Read the model definition and answer for the solid it produces. Units are mm, in the model's axes. A direction names the side the tool comes from. Coordinates: 2 decimals unless noted, no trailing zeros. Write each loop counter-clockwise with the first axis right and the second up, starting at its lowest first coordinate (ties: lowest second). Pieces come first, ordered by that corner, then holes. Notation, with made-up numbers: (-15, 55) -> (1, 55) arc R19 ccw to (1, 72) -> close; hole circle Ø5 at (76.25, 55). An arc over 180 degrees is marked (long way). Write item = value, one per line. Start each with the question number.
1) For a pull along Z with two mould halves and no side action, classify faces 3 (the face through (225, -9, 114.3)), 4 (the face through (196.875, -9.658, 51.917)), 5 (the face through (135, -9, 0)) as released by +Z, released by -Z, zero draft, split by the parting line, or undercut.
2) A tool of negligible diameter and unlimited length cuts with its end or side. For faces 1 (the face through (136, -10, 50.8)), 2 (the face through (273.05, -9, 56)), from which of +Z, -Z, +X, -X, +Y, -Y can it reach the whole face along a straight path? Write none if from no direction.
3) Find the intervals of material crossed by line 1 along Z through (x, y) = (222.25, -9.5); line 2 along X through (y, z) = (-10.25, 106.5); line 3 along X through (y, z) = (-11, 37.5), in increasing order. Write a range as from..to.
4) Flat-ended cylindrical pins translate along their axes: pin 1 Ø4 at (x, y) = (189.5, -2.5) entering from -Z; pin 2 Ø9.5 at (x, y) = (123, -10.5) entering from +Z. Find the tip coordinate at first contact, or state that the pin passes through.
5) Section B-B (y = -14) is taken. Determine the outline of the cut face in (x, z) (3 decimals).
6) Section D-D (z = 30) is taken. Determine the outline of the cut face in (x, y).
7) Section A-A (x = 222.25) is taken. Determine the outline of the cut face in (y, z).
8) Section C-C (z = 85) is taken. Determine the outline of the cut face in (x, y), plus the area to 3 significant figures.
from build123d import *

# Parameters (mm, degrees)
F0_W     = 273.05
F0_H     = 114.3
F1_DEPTH = 19.05
F2_R     = 25.4
F3_DEPTH = 25.4
F5_DEPTH = 25.4


with BuildPart() as f1:
    # F0 (on Front) → F1 (new body)
    with BuildSketch(Plane.XZ):
        with Locations((136.525, 57.15)):
            Rectangle(F0_W, F0_H)
    extrude(amount=F1_DEPTH)

    # F2 (on face) → F3 (cut)
    with BuildSketch(Plane.XZ.offset(19.05)):
        with Locations((50.8, 50.8)):
            Circle(F2_R)
        with Locations((222.25, 50.8)):
            Circle(F2_R)
    extrude(amount=-F3_DEPTH, mode=Mode.SUBTRACT)

    # F4 (on face) → F5 (cut)
    with BuildSketch(Plane.XZ.offset(19.05)):
        with BuildLine():
            Line((177.8, 114.3), (95.25, 114.3))
            Line((95.25, 114.3), (95.25, 60.325))
            ThreePointArc((95.25, 60.325), (98.039808, 53.589808), (104.775, 50.8))
            Line((104.775, 50.8), (168.275, 50.8))
            ThreePointArc((168.275, 50.8), (175.010192, 53.589808), (177.8, 60.325))
            Line((177.8, 60.325), (177.8, 114.3))
        make_face()
    extrude(amount=-F5_DEPTH, mode=Mode.SUBTRACT)


solid = f1.part
Answer key:
q1.face_3 = released by +Z
q1.face_4 = undercut
q1.face_5 = released by -Z
q2.face_1 = +Z, +Y, -Y
q2.face_2 = +Z, -Z, +X, +Y, -Y
q3.line_1 = 0..25.4, 76.2..114.3
q3.line_2 = 0..95.25, 177.8..273.05
q3.line_3 = 0..29.16, 72.44..200.61, 243.89..273.05
q4.pin_1 = 0
q4.pin_2 = 50.8
q5.outline = (0, 0) -> (273.05, 0) -> (273.05, 114.3) -> (177.8, 114.3) -> (177.8, 60.325) arc R9.525 cw to (168.275, 50.8) -> (104.775, 50.8) arc R9.525 cw to (95.25, 60.325) -> (95.25, 114.3) -> (0, 114.3) -> close; hole circle Ø50.8 at (50.8, 50.8); hole circle Ø50.8 at (222.25, 50.8)
q6.outline = (0, -19.05) -> (36.22, -19.05) -> (36.22, 0) -> (0, 0) -> close; (65.38, -19.05) -> (207.67, -19.05) -> (207.67, 0) -> (65.38, 0) -> close; (236.83, -19.05) -> (273.05, -19.05) -> (273.05, 0) -> (236.83, 0) -> close
q7.outline = (-19.05, 0) -> (0, 0) -> (0, 25.4) -> (-19.05, 25.4) -> close; (-19.05, 76.2) -> (0, 76.2) -> (0, 114.3) -> (-19.05, 114.3) -> close
q8.outline = (0, -19.05) -> (95.25, -19.05) -> (95.25, 0) -> (0, 0) -> close; (177.8, -19.05) -> (273.05, -19.05) -> (273.05, 0) -> (177.8, 0) -> close
q8.area = 3,630 mm^2
